CAD build for the part. Positions are in the model's coordinates, mm. Face numbers are marked on the shaded views. A direction names the side the tool comes from. Give positions to 0.01 mm unless a question says otherwise; leave off trailing zeros. Order: outer loops, then holes, each group sorted by start corner. A loop starts at its lowest first (then second) coordinate and runs counter-clockwise, first axis right, second up. Notation, with made-up numbers: (82.25, 86) -> (126.25, 86) arc R17 cw to (126.25, 109) -> close; hole circle Ø1 at (66, -15). An arc over 180 degrees is marked (long way). Answer as CSV lines item,"result".
Autodesk Inventor part; units mm, degrees
ref_plane "Work Plane1" through (0, 74.168, 0) normal (0, 1, 0) x (-1, 0, 0)
ref_plane "YZ Plane" through (0, 0, 0) normal (1, 0, 0) x (0, 1, 0)
ref_plane "XZ Plane" through (0, 0, 0) normal (0, 1, 0) x (-1, 0, 0)
sketch "Sketch2" plane through (0, 0, 0) normal (0, 1, 0) x (-1, 0, 0)
  circle A0 centre (0, 0) radius 1.9812
  dimension "d0" = 3.9624
extrude "Extrusion1" add sketch "Sketch2" along normal blind 50.8
chamfer "Chamfer1" distance 0.7937 angle 45 1 edges at (1.9812, 0, 0)
sketch "Sketch3" plane through (0, 50.8, 0) normal (0, 1, 0) x (1, 0, 0)
  circle A0 centre (0, 0) radius 1.9812
  circle A1 centre (0, 0) radius 4.445
  dimension "d6" = 8.89
extrude "Extrusion2" add sketch "Sketch3" along normal blind 8.89 contours A0 | A1
sketch "Sketch4" plane through (0, 59.69, 0) normal (0, 1, 0) x (1, 0, 0)
  circle A0 centre (0, 0) radius 4.445
  circle A1 centre (0, 0) radius 8.509
  dimension "d9" = 17.018
extrude "Extrusion3" add sketch "Sketch4" along normal blind 2.54 contours A0 | A1
sketch "Sketch5" plane through (0, 0, 0) normal (1, 0, 0) x (0, 1, 0)
  circle A0 centre (68.707, 0) radius 2.667
  arc A1 (70.7539, -5.0629) -> (70.7539, 5.0629) centre (68.707, 0) ccw
  line L0 (59.69, 8.509) -> (62.23, 8.509)
  line L1 (62.23, 8.509) -> (62.23, -8.509)
  line L2 (59.69, -8.509) -> (62.23, -8.509)
  line L3 (62.23, 8.509) -> (62.23, -8.509)
  line L4 (62.23, -8.509) -> (70.7539, -5.0629)
  line L5 (62.23, 8.509) -> (70.7539, 5.0629)
  line L6 (37.7029, 0) -> (42.6845, 0) construction
  line L7 (74.168, 5.5293) -> (74.168, -0.3965) construction
  point P0 (0, 0)
  dimension "d12" = 5.334
  dimension "d13" = 10.922
  dimension "d14" = 11.938
extrude "Extrusion4" add sketch "Sketch5" along normal mid plane 6.096
sketch "Sketch6" plane through (0, 62.23, 0) normal (0, 1, 0) x (1, 0, 0)
  arc A0 (3.048, -7.9444) -> (3.048, 7.9444) centre (0, 0) ccw
  circle A1 centre (0, 0) radius 8.509
  circle A2 centre (0, 0) radius 9.0384
  point P0 (-3.048, 8.509)
extrude "Extrusion5" cut sketch "Sketch6" along normal blind 12.7
sketch "Sketch7" plane through (0, 59.69, 0) normal (0, -1, 0) x (1, 0, 0)
  circle A0 centre (0, 0) radius 8.509
  circle A1 centre (0, 0) radius 4.445
  arc A2 (-4.3273, 1.016) -> (-4.3273, -1.016) centre (0, 0) ccw
  circle A3 centre (0, 0) radius 4.445
  arc A4 (-6.2682, 1.016) -> (-6.2682, -1.016) centre (0, 0) ccw
  line L0 (-6.2682, 1.016) -> (-4.3273, 1.016)
  line L1 (-6.2682, -1.016) -> (-4.3273, -1.016)
  arc A5 (-1.016, -4.3273) -> (1.016, -4.3273) centre (0, 0) ccw
  arc A6 (-1.016, -6.2682) -> (1.016, -6.2682) centre (0, 0) ccw
  line L2 (-1.016, -6.2682) -> (-1.016, -4.3273)
  line L3 (1.016, -6.2682) -> (1.016, -4.3273)
  arc A7 (4.3273, -1.016) -> (4.3273, 1.016) centre (0, 0) ccw
  arc A8 (6.2682, -1.016) -> (6.2682, 1.016) centre (0, 0) ccw
  line L4 (6.2682, -1.016) -> (4.3273, -1.016)
  line L5 (6.2682, 1.016) -> (4.3273, 1.016)
  arc A9 (1.016, 4.3273) -> (-1.016, 4.3273) centre (0, 0) ccw
  arc A10 (1.016, 6.2682) -> (-1.016, 6.2682) centre (0, 0) ccw
  line L6 (1.016, 6.2682) -> (1.016, 4.3273)
  line L7 (-1.016, 6.2682) -> (-1.016, 4.3273)
  dimension "d19" = 12.7
  dimension "d20" = 2.032
  dimension "d21" = 1.016
  dimension "d24" = 360
extrude "Extrusion6" add sketch "Sketch7" along normal blind 8.89 contours A1 L5 A8 L4 | A1 L7 A10 L6 | L3 A6 L2 A1 | A1 L1 A4 L0
ref_plane "Work Plane1" through (0, 74.168, 0) normal (0, 1, 0) x (-1, 0, 0)
properties part number "Shock Mount - Top"
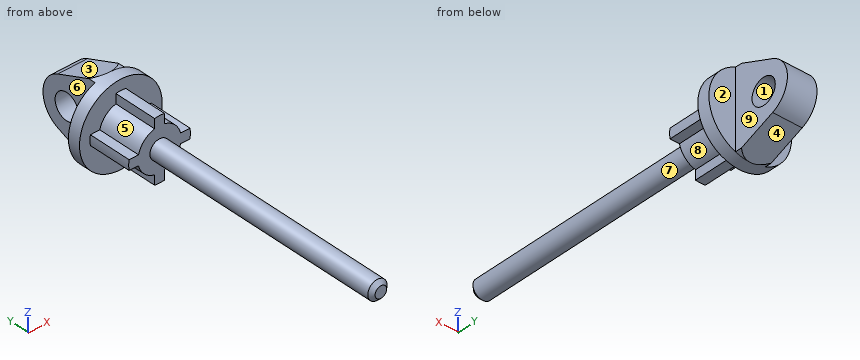
1) Band-saw the part on A-A, the plane z = 0. Write the cut outline in (x, y).
Data:
outline,"(-8.51, 59.69) -> (-6.35, 59.69) -> (-6.35, 50.8) -> (-1.98, 50.8) -> (-1.98, 0.79) -> (-1.19, 0) -> (1.19, 0) -> (1.98, 0.79) -> (1.98, 50.8) -> (6.35, 50.8) -> (6.35, 59.69) -> (8.51, 59.69) -> (8.51, 62.23) -> (3.05, 62.23) -> (3.05, 66.04) -> (-3.05, 66.04) -> (-3.05, 62.23) -> (-8.51, 62.23) -> close; (-3.05, 71.37) -> (3.05, 71.37) -> (3.05, 74.17) -> (-3.05, 74.17) -> close"
2) Wall check: line 1 along Z through (x, y) = (0.25, 56); line 2 along Y through (x, z) = (-6, -3.5); line 3 along Z through (x, y) = (-2.5, 67). Give the ranges that are in metal, low to high. Write a range as [from, to].
Data:
line 1,"z = [-6.35, 6.35]"
line 2,"y = [59.69, 62.23]"
line 3,"z = [-6.58, -2.05], [2.05, 6.58]"
3) Which spindle directions (+Z, -Z, +X, -X, +Y, -Y) get a long thin tool onto all of the face, cutting with end or side? Do the marked faces 5, 6, 7, 8 and 9. Say none if no direction does.
Data:
face 5,"+Z, -X, -Y"
face 6,"+Z, -Z, -X, +Y"
face 7,"-Y"
face 8,"-Z, +X, -Y"
face 9,"+Z, -Z, +X, +Y"
4) Pin check, flat tips, straight feed: P1, Ø6, axis at y = 68.707, z = 0, coming from the -X side; P2, Ø1, axis at x = -2.5, z = -4, coming from the -Y side; P3, Ø1.6, axis at y = 55.5, z = 5.5, coming from the +X side. Stop position of each tip, or through.
Data:
P1,"stops at x = -3.05"
P2,"stops at y = 50.8"
P3,"stops at x = 1.02"
5) Pull direction Z, two halves, no side cores. Call the marked faces 1, 2, 3 and 4: pulls with the +Z half, pulls with the -Z half, needs draft (parallel to the pull), parting line crosses it, or undercut.
Data:
face 1,"undercut"
face 2,"needs draft"
face 3,"pulls with the +Z half"
face 4,"pulls with the -Z half"
6) Band-saw the part on B-B, the plane y = 69. Write the cut outline in (x, z).
Data:
outline,"(-3.05, -5.77) -> (3.05, -5.77) -> (3.05, -2.65) -> (-3.05, -2.65) -> close; (-3.05, 2.65) -> (3.05, 2.65) -> (3.05, 5.77) -> (-3.05, 5.77) -> close"
7) Band-saw the part on C-C, the plane z = -3.5. Write the cut outline in (x, y).
Data:
outline,"(-7.76, 59.69) -> (-2.74, 59.69) -> (-2.74, 50.8) -> (2.74, 50.8) -> (2.74, 59.69) -> (7.76, 59.69) -> (7.76, 62.23) -> (3.05, 62.23) -> (3.05, 72.9) -> (-3.05, 72.9) -> (-3.05, 62.23) -> (-7.76, 62.23) -> close"
8) Band-saw the part on D-D, the plane x = 7.25. Write the cut outline in (y, z), then the cut area to 3 significant figures.
Data:
outline,"(59.69, -4.45) -> (62.23, -4.45) -> (62.23, 4.45) -> (59.69, 4.45) -> close"
area,"22.6 mm2"
